Geometry: see drawing. Coordinates: mm, zero at the bounding-box minimum. A direction names the side the tool comes from. Give positions to 0.01 mm unless a question says otherwise; leave off trailing zeros. Write each loop counter-clockwise with the first axis right and the second up, starting at its lowest first coordinate (ties: lowest second). Pieces come first, ordered by that corner, then holes. Notation, with made-up numbers: (6.25, -5) -> (51.25, -5) arc R32 ccw to (51.25, 32) -> close; hole circle Ø3 at (-11, 40.25). An arc over 180 degrees is marked (long way). Use one line per item in the form item = value. Start each with the question number.
(1) First-contact query: P1, Ø3.5, axis at y = 63, z = 21, coming from the +X side; P2, Ø9.5, axis at x = 19, y = 32.5, coming from the +Z side; P3, Ø5, axis at x = 16, y = 55, coming from the +Z side. Flat tips, straight axial feed; report the tip coordinate or a pass-through.
(2) Material intervals for line 1 along X through (y, z) = (21.5, 20); line 2 along X through (y, z) = (82.5, 38.5), sorted ascending. Write a range as from..to.
(3) Cut plane B-B, the plane z = 3.5. Output: boundary loops of the cut face in (x, y).
(4) Draft query along X for the marked faces 1, 2, 3 and 4. Return one class per face: pulls with the +X half, pulls with the -X half, needs draft (parallel to the pull), parting line crosses it, or undercut.
(5) Cut plane A-A, the plane x = 20. Output: boundary loops of the cut face in (y, z), and give its area (3 significant figures).
(6) Set-up query: the marked faces 5, 6, 7, 8 and 9. Return all of +Z, -Z, +X, -X, +Y, -Y with unobstructed straight access to the full face (end or side cutting, diameter ignored); none if empty.
(7) Cut plane C-C, the plane z = 10.5. Output: boundary loops of the cut face in (x, y).
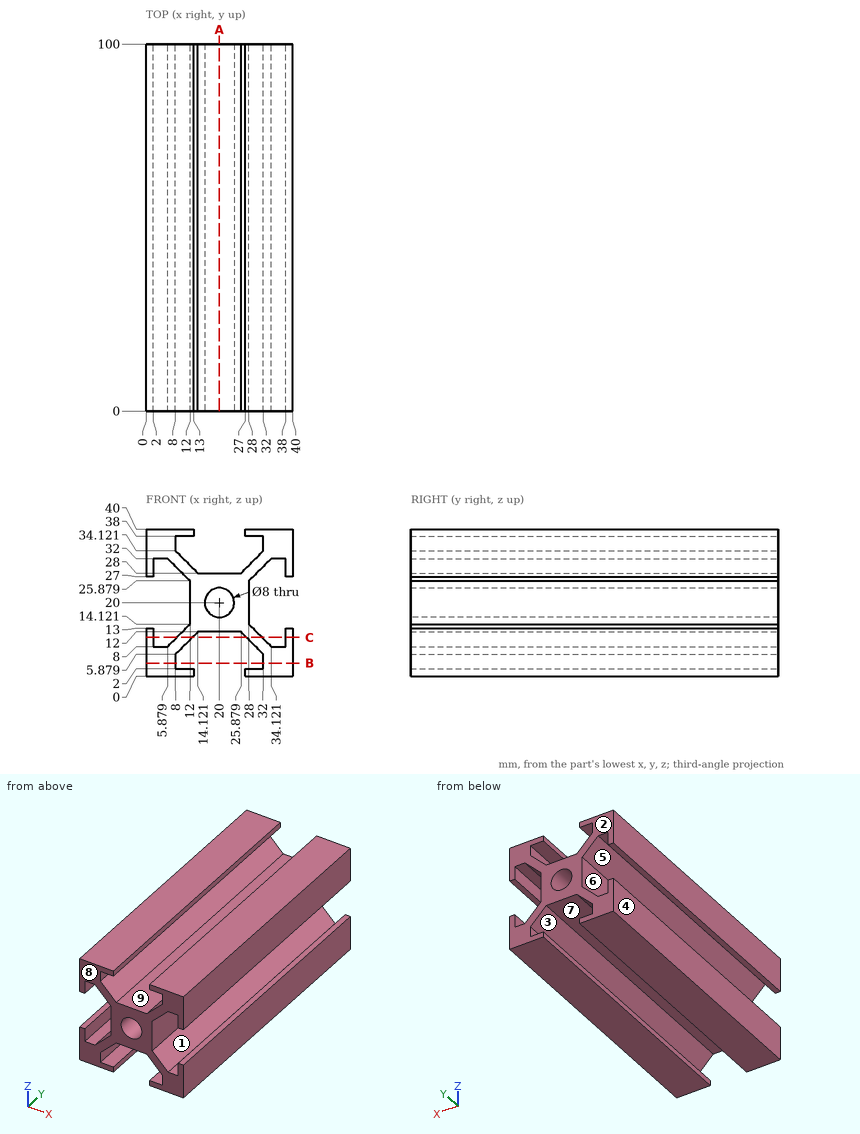
Geometry says:
q1.P1 = 28
q1.P2 = 28
q1.P3 = 28.62
q2.line_1 = 12..16, 24..28
q2.line_2 = 0..13, 27..40
q3.outline = (0, 0) -> (8, 0) -> (8, 100) -> (0, 100) -> close; (32, 0) -> (40, 0) -> (40, 100) -> (32, 100) -> close
q4.face_1 = undercut
q4.face_2 = needs draft
q4.face_3 = undercut
q4.face_4 = pulls with the -X half
q5.outline = (0, 12) -> (100, 12) -> (100, 16) -> (0, 16) -> close; (0, 24) -> (100, 24) -> (100, 28) -> (0, 28) -> close
q5.area = 800 mm^2
q6.face_5 = +Y, -Y
q6.face_6 = -X, +Y, -Y
q6.face_7 = -Z, +Y, -Y
q6.face_8 = +Z, -Z, +X, -X, -Y
q6.face_9 = +Z, +Y, -Y
q7.outline = (0, 0) -> (2, 0) -> (2, 100) -> (0, 100) -> close; (8.38, 0) -> (12.62, 0) -> (12.62, 100) -> (8.38, 100) -> close; (27.38, 0) -> (31.62, 0) -> (31.62, 100) -> (27.38, 100) -> close; (38, 0) -> (40, 0) -> (40, 100) -> (38, 100) -> close
